```python
from build123d import *

# Parameters (mm, degrees)
SKETCH1_W           = 109.52
SKETCH1_H           = 90
BOSS_EXTRUDE1_DEPTH = 5
SKETCH2_R           = 0.95
CUT_EXTRUDE1_DEPTH  = 7
FILLET1_R           = 3
BOSS_EXTRUDE2_DEPTH = 3.5
CHAMFER1_SIZE       = 3.5
CHAMFER1_SIZE2      = 4.171137574
SKETCH5_W           = 100.2
SKETCH5_H           = 79.2
CUT_EXTRUDE3_DEPTH  = 6.5
SKETCH8_R           = 1.45
CUT_EXTRUDE5_DEPTH  = 3


with BuildPart() as part:
    # Sketch1 → Boss-Extrude1 (new body)
    with BuildSketch(Plane.XY):
        with Locations((49.453432203, -35.801949153)):
            Rectangle(SKETCH1_W, SKETCH1_H)
    extrude(amount=BOSS_EXTRUDE1_DEPTH)

    # Sketch2 → Cut-Extrude1 (cut)
    with BuildSketch(Plane(origin=(0, 9.198050847, 0), x_dir=(1, 0, 0), z_dir=(0, 1, 0))):
        with Locations(Location((-3.306567797, -2.5, 0), (0, 0, 270))):
            Circle(SKETCH2_R)
        with Locations(Location((102.213432203, -2.5, 0), (0, 0, 270))):
            Circle(SKETCH2_R)
    extrude(amount=-CUT_EXTRUDE1_DEPTH, mode=Mode.SUBTRACT)

    # Fillet1
    fillet1_edges = [part.edges().sort_by_distance(p)[0] for p in [
        (104.213432203, -80.801949153, 2.5),
        (-5.306567797, -80.801949153, 2.5),
    ]]
    fillet(fillet1_edges, radius=FILLET1_R)

    # Sketch4 → Boss-Extrude2 (add)
    with BuildSketch(Plane(origin=(0, 0, 0), x_dir=(-1, 0, 0), z_dir=(0, 0, -1))):
        with BuildLine():
            Line((-104.213432203, 9.198050847), (-104.213432203, -77.801949153))
            ThreePointArc((-104.213432203, -77.801949153), (-103.334752547, -79.923269496), (-101.213432203, -80.801949153))
            Line((-101.213432203, -80.801949153), (2.306567797, -80.801949153))
            ThreePointArc((2.306567797, -80.801949153), (4.42788814, -79.923269496), (5.306567797, -77.801949153))
            Line((5.306567797, -77.801949153), (5.306567797, 9.198050847))
            Line((5.306567797, 9.198050847), (-104.213432203, 9.198050847))
        make_face()
    extrude(amount=BOSS_EXTRUDE2_DEPTH)

    # Chamfer1
    chamfer1_edges = [part.edges().sort_by_distance(p)[0] for p in [
        (49.453432203, 9.198050847, -3.5),
    ]]
    chamfer1_side = [part.faces().sort_by_distance(p)[0] for p in [
        (49.453432203, 9.198050847, 0.739274778),
    ]]
    chamfer(chamfer1_edges, length=CHAMFER1_SIZE, length2=CHAMFER1_SIZE2, reference=chamfer1_side[0])

    # Sketch5 → Cut-Extrude3 (cut)
    with BuildSketch(Plane(origin=(0, 0, -3.5), x_dir=(-1, 0, 0), z_dir=(0, 0, -1))):
        with Locations((-49.453432203, -35.801949153)):
            Rectangle(SKETCH5_W, SKETCH5_H)
    extrude(amount=-CUT_EXTRUDE3_DEPTH, mode=Mode.SUBTRACT)

    # Sketch8 → Cut-Extrude5 (cut)
    with BuildSketch(Plane(origin=(104.213432203, 0, 0), x_dir=(0, 0, -1), z_dir=(1, 0, 0))):
        with Locations((0.5, -66.551949153)):
            Circle(SKETCH8_R)
    cut_extrude5 = extrude(amount=-CUT_EXTRUDE5_DEPTH, mode=Mode.SUBTRACT)

    # Mirror2: Cut-Extrude5 across plane
    add(cut_extrude5.mirror(Plane.ZY.offset(-49.453432203)), mode=Mode.SUBTRACT)


solid = part.part
```
Here's how the part is built. I have some questions about the finished solid (model axes, mm). A direction names the side the tool comes from. Give positions to 0.01 mm unless a question says otherwise; leave off trailing zeros. Order: outer loops, then holes, each group sorted by start corner. A loop starts at its lowest first (then second) coordinate and runs counter-clockwise, first axis right, second up. Notation, with made-up numbers: (89, 66) - (135, 66) arc R24 cw to (135, 96) - close; hole circle Ø8 at (73.25, 66). An arc over 180 degrees is marked (long way). Answer as a JSON object with one key per item and string values. Group by question number.
Item 1: Please list where these lines run through material, in increasing order: probe 1 along X at (y, z) = (5, 2.5); probe 2 along X at (y, z) = (-2, 0.75); probe 3 along Y at (x, z) = (35, 2.5).
Item 2: If we section it at A-A on x = 51: Please give me the cut outline in (y, z), and give its area (3 significant figures).
Item 3: If we mould it in two halves opening along Y, with no side actions, what happens to faces 4 (the flat face through (-5.307, -35, 1)), 5 (the flat face through (-0.647, -36, 0)), 6 (the flat face through (50, 3.798, 0)), 7 (the flat face through (49, 9.198, 3))? For each: pulls with the +Y half, pulls with the -Y half, needs draft (parallel to the pull), parting line crosses it, or undercut.
Item 4: Which directions (+Z, -Z, +X, -X, +Y, -Y) give clear straight access to the entire face, cutting with the end or side of a thin tool? Please do faces 1 (the flat face through (50, -75.402, 0)), 2 (the flat face through (101.213, -67, 0)), 3 (the flat face through (-2.307, -67, 0)).
Item 5: For P1, Ø8, axis at x = 35, y = -55, coming from the -Z side; P2, Ø2.5, axis at y = -66.55, z = -0.5, coming from the -X side; P3, Ø1.5, axis at x = -3.31, z = 2.5, coming from the +Y side, each with a flat end and sliding along its axis, tell me the tip position at first contact or that it passes through.
Item 6: If we section it at B-B on y = -12.5: Please give me the cut outline in (x, z), and give its area (3 significant figures).
Result set:
{
 "1": {"probe 1": "-5.31 to -4.26, -2.36 to 101.26, 103.16 to 104.21", "probe 2": "-5.31 to -0.65, 99.55 to 104.21", "probe 3": "-80.8 to -75.4, 3.8 to 9.2"},
 "2": {"outline": "(-80.8, -3.5) - (-75.4, -3.5) - (-75.4, 3) - (3.8, 3) - (3.8, -3.5) - (5.03, -3.5) - (9.2, 0) - (9.2, 5) - (-80.8, 5) - close", "area": "243 mm²"},
 "3": {"face 4": "needs draft", "face 5": "undercut", "face 6": "undercut", "face 7": "pulls with the +Y half"},
 "4": {"face 1": "-Z", "face 2": "+X", "face 3": "-X"},
 "5": {"P1": "z = 3", "P2": "x = -2.31", "P3": "y = 2.2"},
 "6": {"outline": "(-5.31, -3.5) - (-0.65, -3.5) - (-0.65, 3) - (99.55, 3) - (99.55, -3.5) - (104.21, -3.5) - (104.21, 5) - (-5.31, 5) - close", "area": "280 mm²"}
}
